Input: part model. Units: mm. Frame: model coordinates. Face numbers are marked on the shaded views. A direction names the side the tool comes from. Round coordinates to 2 decimals unless told otherwise and drop trailing zeros. Order: outer loops, then holes, each group sorted by start corner. A loop starts at its lowest first (then second) coordinate and runs counter-clockwise, first axis right, second up. Notation, with made-up numbers: (79.25, 10.5) -> (132.25, 10.5) arc R17 ccw to (132.25, 22.5) -> close; hole circle Ø8 at (26.5, 67). An arc over 180 degrees is marked (long way). Answer as CSV lines item,"result". Start each with the question number.
1) Section query C-C, the plane y = 12. Output: boundary loops of the cut face in (x, z), and give its area (3 significant figures).
2) Section query B-B, the plane x = 8.5. Output: boundary loops of the cut face in (y, z), and give its area (3 significant figures).
3) Access query for the marked faces 4, 5, 6 and 7. Directions: +Z, -Z, +X, -X, +Y, -Y. A direction counts if a zero-diameter tool reaches every point of the face in a straight line with its end or side. Return the directions, or none.
4) Section query A-A, the plane z = -7. Output: boundary loops of the cut face in (x, y).
5) Mould query, pull axis Y, two halves, no side actions, for the marked faces 1, 2 and 3. Classes: +Y half, -Y half, draft (parallel to the pull), parting line (faces both ways), or undercut.
6) Section query D-D, the plane x = 19.25. Output: boundary loops of the cut face in (y, z).
7) Line query: L1, parallel to Z at x = 11, y = 12.5; L2, parallel to Y at x = 17.75, z = -19.5; L3, parallel to Y at x = 11.75, z = -8.25. Output: solid intervals per line, ascending.
8) First-contact query: P1, Ø1, axis at x = 12.5, z = -14, coming from the +Y side; P2, Ø10, axis at x = 11, z = -9, coming from the -Y side; P3, Ø6.5, axis at x = 9.5, y = 9, coming from the +Z side; P4, Ø2.5, axis at y = 7, z = -12.5, coming from the +X side. Flat tips, straight axial feed; report the tip coordinate or a pass-through.
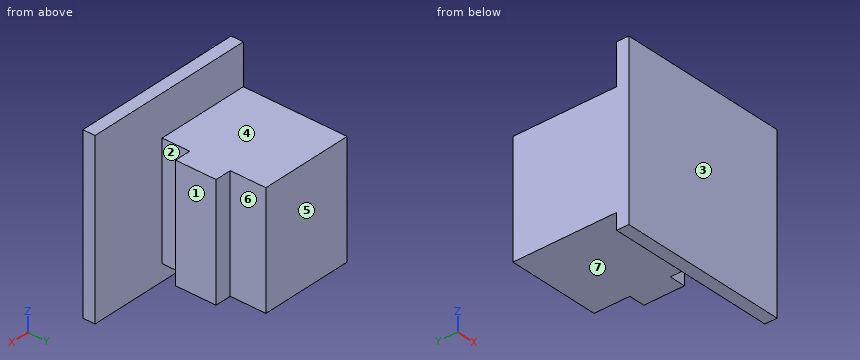
```python
from build123d import *

# Parameters (mm, degrees)
SKETCH1_W           = 21
SKETCH1_H           = 21
BOSS_EXTRUDE1_DEPTH = 1.5
BOSS_EXTRUDE3_DEPTH = 14


with BuildPart() as part:
    # Sketch1 → Boss-Extrude1 (new body)
    with BuildSketch(Plane(origin=(0, 0, 0), x_dir=(1, 0, 0), z_dir=(0, 1, 0))):
        with Locations((10.5, 10.5)):
            Rectangle(SKETCH1_W, SKETCH1_H)
    extrude(amount=BOSS_EXTRUDE1_DEPTH)

    # Sketch3 → Boss-Extrude3 (add)
    with BuildSketch(Plane(origin=(0, 0, -19), x_dir=(-1, 0, 0), z_dir=(0, 0, -1))):
        Polygon((0, 1.5), (0, 14.3), (-11.5, 14.3), (-11.5, 9.9), (-13.5, 9.9), (-13.5, 4.9), (-11.5, 4.9), (-11.5, 1.5), align=None)
    extrude(amount=-BOSS_EXTRUDE3_DEPTH)


solid = part.part
```
Findings:
1,outline,"(0, -19) -> (11.5, -19) -> (11.5, -5) -> (0, -5) -> close"
1,area,"161 mm^2"
2,outline,"(0, -21) -> (1.5, -21) -> (1.5, -19) -> (14.3, -19) -> (14.3, -5) -> (1.5, -5) -> (1.5, 0) -> (0, 0) -> close"
2,area,"211 mm^2"
3,face 4,"+Z, +X, -X, +Y"
3,face 5,"+Z, -Z, +X, -X, +Y"
3,face 6,"+Z, -Z, +X, +Y"
3,face 7,"-Z, +X, -X, +Y"
4,outline,"(0, 0) -> (21, 0) -> (21, 1.5) -> (11.5, 1.5) -> (11.5, 4.9) -> (13.5, 4.9) -> (13.5, 9.9) -> (11.5, 9.9) -> (11.5, 14.3) -> (0, 14.3) -> close"
5,face 1,"draft"
5,face 2,"undercut"
5,face 3,"-Y half"
6,outline,"(0, -21) -> (1.5, -21) -> (1.5, 0) -> (0, 0) -> close"
7,L1,"z = -19 to -5"
7,L2,"y = 0 to 1.5"
7,L3,"y = 0 to 1.5, 4.9 to 9.9"
8,P1,"stops at y = 9.9"
8,P2,"stops at y = 0"
8,P3,"stops at z = -5"
8,P4,"stops at x = 13.5"
